Could you check a few things on this model? Use its own coordinates, in mm. Give positions to 0.01 mm unless a question says otherwise; leave off trailing zeros. Write each loop counter-clockwise with the first axis right and the second up, starting at its lowest first coordinate (ties: lowest second). Pieces come first, ordered by that corner, then holes. Notation, with made-up numbers: (11.25, -38) - (31.25, -38) arc R25 cw to (31.25, -22) - close; hole circle Ø8 at (14.25, -10). An arc over 180 degrees is marked (long way). Answer in a Markdown table with one row per item.
from build123d import *

# Parameters (mm, degrees)
F1_DEPTH = 150
F3_D     = 30
F4_R     = 15
F5_DEPTH = 150


with BuildPart() as f1:
    # F0 (on Front) → F1 (new body)
    with BuildSketch(Plane.XZ):
        with BuildLine():
            ThreePointArc((75, 55), (69.142136, 69.142136), (55, 75))
            Line((55, 75), (-55, 75))
            ThreePointArc((-55, 75), (-69.142136, 69.142136), (-75, 55))
            Line((-75, 55), (-75, -55))
            ThreePointArc((-75, -55), (-69.142136, -69.142136), (-55, -75))
            Line((-55, -75), (55, -75))
            ThreePointArc((55, -75), (69.142136, -69.142136), (75, -55))
            Line((75, -55), (75, 55))
        make_face()
    extrude(amount=F1_DEPTH)

    # F3 (through all)
    with Locations(Plane.XZ.offset(150)):
        with Locations((3.283451, 8.47559)):
            Hole(F3_D / 2)

    # F4 (on face) → F5 (cut)
    with BuildSketch(Plane.YZ.offset(75)):
        with Locations((-75, 0)):
            Circle(F4_R)
    extrude(amount=-F5_DEPTH, mode=Mode.SUBTRACT)


solid = f1.part
1) If I drill on line 1 (Y direction, x = -34, z = 0); line 2 (Z direction, x = -4, y = -126.5); line 3 (Z direction, x = -24.5, y = -64), over which ranges is the centre line in solid material (lowest first)?
Check values:
| item | result |
|---|---|
| line 1 | y = -150 to -90, -60 to 0 |
| line 2 | z = -75 to -4.64, 21.59 to 75 |
| line 3 | z = -75 to -10.2, 10.2 to 75 |
2) Imagine slicing it at B-B (x = 45). List the corners of the cut face in (y, z) for me.
Check values:
| item | result |
|---|---|
| outline | (-150, -75) - (0, -75) - (0, 75) - (-150, 75) - close; hole circle Ø30 at (-75, 0) |
3) We'd pull the mould along Z, two halves only. Please class faces 1 (the face through (5.236, -73.95, 23.348)), 2 (the face through (1.05, -78.252, -14.643)), 3 (the face through (75, -91, -1)), 4 (the face through (-69.297, -73.95, -68.986)): +Z half, -Z half, draft (parallel to the pull), parting line (faces both ways), or undercut.
Check values:
| item | result |
|---|---|
| face 1 | undercut |
| face 2 | undercut |
| face 3 | draft |
| face 4 | -Z half |
4) Imagine slicing it at A-A (y = -72). List the corners of the cut face in (x, z) for me.
Check values:
| item | result |
|---|---|
| outline | (-75, -55) arc R20 ccw to (-55, -75) - (55, -75) arc R20 ccw to (75, -55) - (75, -14.7) - (-75, -14.7) - close; (-75, 14.7) - (-10.37, 14.7) arc R15 cw to (16.93, 14.7) - (75, 14.7) - (75, 55) arc R20 ccw to (55, 75) - (-55, 75) arc R20 ccw to (-75, 55) - close |
5) Imagine slicing it at D-D (z = 0). List the corners of the cut face in (x, y) for me, then the cut area to 3 significant figures.
Check values:
| item | result |
|---|---|
| outline | (-75, -150) - (-9.09, -150) - (-9.09, -90) - (-75, -90) - close; (-75, -60) - (-9.09, -60) - (-9.09, 0) - (-75, 0) - close; (15.66, -150) - (75, -150) - (75, -90) - (15.66, -90) - close; (15.66, -60) - (75, -60) - (75, 0) - (15.66, 0) - close |
| area | 15,000 mm2 |
6) Imagine slicing it at C-C (x = 8). List the corners of the cut face in (y, z) for me, then the cut area to 3 significant figures.
Check values:
| item | result |
|---|---|
| outline | (-150, -75) - (0, -75) - (0, -5.76) - (-61.15, -5.76) arc R15 cw to (-88.85, -5.76) - (-150, -5.76) - close; (-150, 22.71) - (0, 22.71) - (0, 75) - (-150, 75) - close |
| area | 18,000 mm2 |
